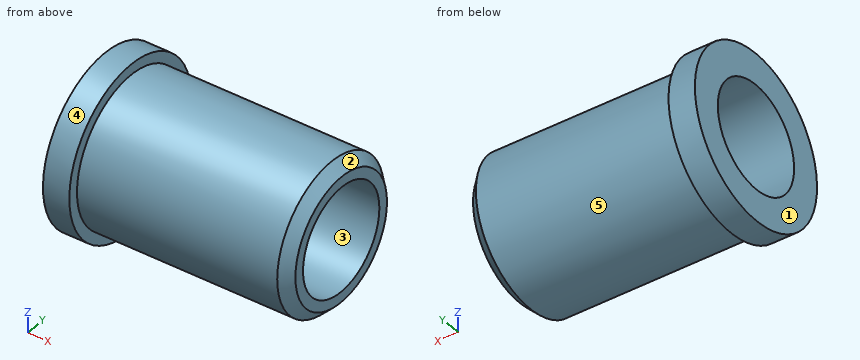
Autodesk Inventor part; units mm, degrees
ref_plane "YZ Plane" through (0, 0, 0) normal (1, 0, 0) x (0, 1, 0)
ref_plane "XZ Plane" through (0, 0, 0) normal (0, 1, 0) x (-1, 0, 0)
ref_plane "XY Plane" through (0, 0, 0) normal (0, 0, 1) x (1, 0, 0)
sketch "Skizze1" plane through (0, 0, 0) normal (1, 0, 0) x (0, 1, 0)
  circle A0 centre (0, 0) radius 14
  circle A1 centre (0, 0) radius 10
  dimension "d0" = 28
  dimension "d1" = 20
extrude "Extrusion1" add sketch "Skizze1" along normal blind 40
chamfer "Fasen1" distance 2 angle 45 1 edges at (40, -14, 0)
sketch "Skizze2" plane through (0, 0, 0) normal (-1, 0, 0) x (0, 0, 1)
  circle A0 centre (0, 0) radius 16
  circle A1 centre (0, 0) radius 10
  dimension "d7" = 32
extrude "Extrusion2" add sketch "Skizze2" along normal blind 5
properties part number "LagerBund" material "Nylon 6/6"
Read the model definition and answer for the solid it produces. Units are mm, in the model's axes. Face numbers are marked on the shaded views. A direction names the side the tool comes from. Coordinates: 2 decimals unless noted, no trailing zeros. Write each loop counter-clockwise with the first axis right and the second up, starting at its lowest first coordinate (ties: lowest second). Pieces come first, ordered by that corner, then holes. Notation, with made-up numbers: (60, 26.5) -> (83, 26.5) arc R28 cw to (83, 64.5) -> close; hole circle Ø11 at (-30, 12). An arc over 180 degrees is marked (long way). Return JSON: item names as keys, results as strings.
(1) Which of the six approach directions +Z, -Z, +X, -X, +Y, -Y give full straight-line access (tool end or side, diameter ignored) to the marked faces 4 and 5?
Answers below:
{"face 4": "+X, -X", "face 5": "+X"}
(2) The part is cut by section A-A on x = 5.5. Give the vertices of the cut face in (y, z), then the cut area to 3 significant figures.
Answers below:
{"outline": "circle Ø28 at (0, 0); hole circle Ø20 at (0, 0)", "area": "302 mm^2"}
(3) Each of these flat-tipped pins is pushed along its axis until it touches: P1, Ø3, axis at x = 17, y = -7.5, coming from the +Z side; P2, Ø3, axis at y = 9, z = 12, coming from the +X side; P3, Ø3, axis at x = 1, y = 10.5, coming from the +Z side. Where does it stop, or does it pass through?
Answers below:
{"P1": "z = 12.65", "P2": "x = 38.5", "P3": "z = 12.96"}
(4) Consider line 1 along Z through (x, y) = (16.5, 0); line 2 along X through (y, z) = (-2.5, -14); line 3 along Y through (x, z) = (8, 2). Determine where each line is inside the solid, lowest interval first. Write a range as from..to.
Answers below:
{"line 1": "-14..-10, 10..14", "line 2": "-5..0", "line 3": "-13.86..-9.8, 9.8..13.86"}
(5) For a pull along Y with two mould halves and no side action, classify the marked faces 1, 2 and 3 as pulls with the +Y half, pulls with the -Y half, needs draft (parallel to the pull), parting line crosses it, or undercut.
Answers below:
{"face 1": "needs draft", "face 2": "parting line crosses it", "face 3": "undercut"}
